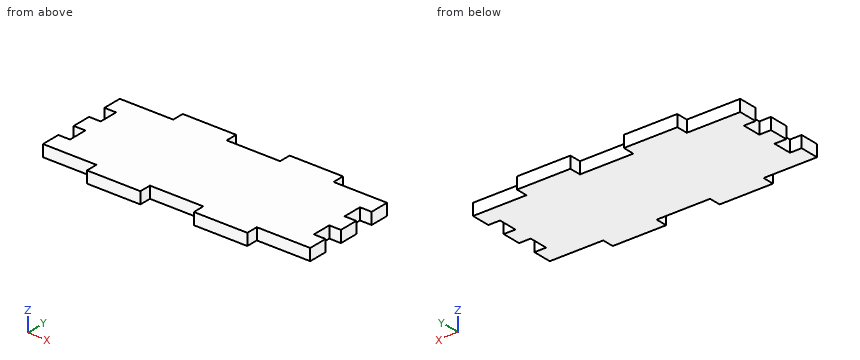
```python
from build123d import *

# Parameters (mm, degrees)
SKETCH3_R           = 4
BOSS_EXTRUDE2_DEPTH = 10


with BuildPart() as part:
    # Sketch3 → Boss-Extrude2 (new body)
    # profile 1 of 5: a face of its own
    with BuildSketch(Plane.XY):
        Polygon((102.429124183, -12.51217232), (56.709124183, -12.51217232), (56.709124183, -22.51217232), (10.989124183, -22.51217232), (10.989124183, -12.51217232), (-24.730875817, -12.51217232), (-34.730875817, -12.51217232), (-34.730875817, 3.64782768), (-24.730875817, 3.64782768), (-24.730875817, 19.80782768), (-34.730875817, 19.80782768), (-34.730875817, 35.96782768), (-24.730875817, 35.96782768), (-24.730875817, 52.12782768), (-34.730875817, 52.12782768), (-34.730875817, 68.28782768), (-24.730875817, 68.28782768), (10.989124183, 68.28782768), (10.989124183, 78.28782768), (56.709124183, 78.28782768), (56.709124183, 68.28782768), (102.429124183, 68.28782768), (102.429124183, 78.28782768), (148.149124183, 78.28782768), (148.149124183, 68.28782768), (183.869124183, 68.28782768), (193.869124183, 68.28782768), (193.869124183, 52.12782768), (183.869124183, 52.12782768), (183.869124183, 35.96782768), (193.869124183, 35.96782768), (193.869124183, 19.80782768), (183.869124183, 19.80782768), (183.869124183, 3.64782768), (193.869124183, 3.64782768), (193.869124183, -12.51217232), (183.869124183, -12.51217232), (148.149124183, -12.51217232), (148.149124183, -22.51217232), (102.429124183, -22.51217232), align=None)
        with Locations((-12.030875817, 55.58782768)):
            Circle(SKETCH3_R, mode=Mode.SUBTRACT)
        with Locations((171.169124183, 55.58782768)):
            Circle(SKETCH3_R, mode=Mode.SUBTRACT)
        with Locations((-12.030875817, 0.18782768)):
            Circle(SKETCH3_R, mode=Mode.SUBTRACT)
        with Locations((171.169124183, 0.18782768)):
            Circle(SKETCH3_R, mode=Mode.SUBTRACT)
    # profile 2 of 5: a face of its own
    with BuildSketch(Plane.XY):
        with Locations((-12.030875817, 55.58782768)):
            Circle(SKETCH3_R)
    # profile 3 of 5: a face of its own
    with BuildSketch(Plane.XY):
        with Locations((-12.030875817, 0.18782768)):
            Circle(SKETCH3_R)
    # profile 4 of 5: a face of its own
    with BuildSketch(Plane.XY):
        with Locations((171.169124183, 0.18782768)):
            Circle(SKETCH3_R)
    # profile 5 of 5: a face of its own
    with BuildSketch(Plane.XY):
        with Locations((171.169124183, 55.58782768)):
            Circle(SKETCH3_R)
    extrude(amount=BOSS_EXTRUDE2_DEPTH)


solid = part.part
```
CAD build for the part. Positions are in the model's coordinates, mm. Coordinates: 2 decimals unless noted, no trailing zeros. Loops run counter-clockwise (first coordinate to the right, second up) from the corner with the lowest first, then second, coordinate; pieces in that order, holes last. Notation, with made-up numbers: (61, 22) - (71, 22) arc R13 ccw to (71, 28) - close; hole circle Ø9 at (31.25, -1.75). An arc over 180 degrees is marked (long way). Return JSON: item names as keys, results as strings.
1. Band-saw the part on B-B (x = 92.5). Give the cut face in (y, z), and give its area (3 significant figures).
Result:
{"outline": "(-12.51, 0) - (68.29, 0) - (68.29, 10) - (-12.51, 10) - close", "area": "808 mm2"}
2. Band-saw the part on A-A (y = 40). Give the cut face in (x, z).
Result:
{"outline": "(-24.73, 0) - (183.87, 0) - (183.87, 10) - (-24.73, 10) - close"}
3. Probe L1, parallel to X at y = 70, z = 7; L2, parallel to Y at x = 70, z = 4; L3, parallel to X at y = 42.5, z = 9.5. List the from-to ranges inside material, lowest first. Write a range as from..to.
Result:
{"L1": "x = 10.99..56.71, 102.43..148.15", "L2": "y = -12.51..68.29", "L3": "x = -24.73..183.87"}
4. Drop flat-ended pins along their axis: pin 1 (5 mm diameter, centred on x = 189.5, z = 5.5, fed in from +Y); pin 2 (5 mm diameter, centred on x = 191, z = 6.5, fed in from -Y); pin 3 (6 mm diameter, centred on y = 43.5, z = 7, fed in from -X). Give the stop position or say it passes through.
Result:
{"pin 1": "stops at y = 68.29", "pin 2": "stops at y = -12.51", "pin 3": "stops at x = -24.73"}
